from build123d import *

# Parameters (mm, degrees)
F1_DEPTH       = 7
F2_DEPTH       = 6
F3_W           = 4.4
F3_H           = 18
F4_DEPTH       = 18
F6_D           = 4.4
F6_DEPTH       = 5
F6_CSINK_D     = 8.96
F6_CSINK_ANGLE = 90
F6_TIP         = 1.3218933619
F8_DEPTH       = 2.6
F9_R           = 2.2
F10_DEPTH      = 2.3


# Not quite as in the source:
# - a pattern or mirror of a feature is missing from the dataset's text; its kind, count and spacing are read off the source's solid


with BuildPart() as f1:
    # F0 (on Front) → F1 (new body, symmetric)
    with BuildSketch(Plane.XZ):
        with BuildLine():
            Line((129.5, 0), (174.5, 0))
            ThreePointArc((174.5, 0), (174.2671322418, 9.0120264206), (173.5691504848, 18))
            ThreePointArc((173.5691504848, 18), (0, 174.5), (-173.5691504848, 18))
            ThreePointArc((-173.5691504848, 18), (-174.2671322418, 9.0120264206), (-174.5, 0))
            Line((-174.5, 0), (-129.5, 0))
            ThreePointArc((-129.5, 0), (0, 129.5), (129.5, 0))
        make_face()
        with BuildLine():
            ThreePointArc((173.5691504848, 18), (174.2671322418, 9.0120264206), (174.5, 0))
            Line((174.5, 0), (194.5, 0))
            Line((194.5, 0), (194.5, 18))
            Line((194.5, 18), (173.5691504848, 18))
        make_face()
        with BuildLine():
            ThreePointArc((-174.5, 0), (-174.2671322418, 9.0120264206), (-173.5691504848, 18))
            Line((-173.5691504848, 18), (-194.5, 18))
            Line((-194.5, 18), (-194.5, 0))
            Line((-194.5, 0), (-174.5, 0))
        make_face()
    extrude(amount=F1_DEPTH, both=True)

    # F0 (on Front) → F2 (join, symmetric)
    with BuildSketch(Plane.XZ):
        with BuildLine():
            Line((129.5, 0), (174.5, 0))
            ThreePointArc((174.5, 0), (174.2671322418, 9.0120264206), (173.5691504848, 18))
            ThreePointArc((173.5691504848, 18), (0, 174.5), (-173.5691504848, 18))
            ThreePointArc((-173.5691504848, 18), (-174.2671322418, 9.0120264206), (-174.5, 0))
            Line((-174.5, 0), (-129.5, 0))
            ThreePointArc((-129.5, 0), (0, 129.5), (129.5, 0))
        make_face()
        with BuildLine():
            ThreePointArc((173.5691504848, 18), (174.2671322418, 9.0120264206), (174.5, 0))
            Line((174.5, 0), (194.5, 0))
            Line((194.5, 0), (194.5, 18))
            Line((194.5, 18), (173.5691504848, 18))
        make_face()
        with BuildLine():
            ThreePointArc((-174.5, 0), (-174.2671322418, 9.0120264206), (-173.5691504848, 18))
            Line((-173.5691504848, 18), (-194.5, 18))
            Line((-194.5, 18), (-194.5, 0))
            Line((-194.5, 0), (-174.5, 0))
        make_face()
    extrude(amount=F2_DEPTH, both=True)

    # F3 (on face) → F4 (cut)
    with BuildSketch(Plane.YZ.offset(194.5)):
        with Locations((0, 9)):
            Rectangle(F3_W, F3_H)
    f4 = extrude(amount=-F4_DEPTH, mode=Mode.SUBTRACT)

    # F4_copies: F4 across plane
    add(f4.mirror(Plane(origin=(0, 0, 0), x_dir=(0, 0, -1), z_dir=(-1, 0, 0))), mode=Mode.SUBTRACT)

    # F6
    with Locations(Plane.XZ.offset(7)):
        with Locations((185.5, 9)):
            f6 = CounterSinkHole(F6_D / 2, F6_CSINK_D / 2, depth=F6_DEPTH, counter_sink_angle=F6_CSINK_ANGLE)
            with Locations((0, 0, -(F6_DEPTH + F6_TIP / 2))):  # 118° drill point
                Cone(0, F6_D / 2, F6_TIP, mode=Mode.SUBTRACT)

    # F6_copies: F6 across plane
    add(f6.mirror(Plane(origin=(0, 0, 0), x_dir=(0, 0, -1), z_dir=(-1, 0, 0))), mode=Mode.SUBTRACT)

    # F7 (on face) → F8 (cut)
    with BuildSketch(Plane(origin=(0, 7, 0), x_dir=(-1, 0, 0), z_dir=(0, 1, 0))):
        Polygon((-189, 11.0207259422), (-189, 6.9792740578), (-185.5, 4.9585481157), (-182, 6.9792740578), (-182, 11.0207259422), (-185.5, 13.0414518843), align=None)
    f8 = extrude(amount=-F8_DEPTH, mode=Mode.SUBTRACT)

    # F8_copies: F8 across plane
    add(f8.mirror(Plane(origin=(0, 0, 0), x_dir=(0, 0, -1), z_dir=(-1, 0, 0))), mode=Mode.SUBTRACT)

    # F9 (on face) → F10 (cut)
    with BuildSketch(Plane(origin=(0, 4.4, 0), x_dir=(-1, 0, 0), z_dir=(0, 1, 0))):
        with Locations((-185.5, 9)):
            Circle(F9_R)
    f10 = extrude(amount=-F10_DEPTH, mode=Mode.SUBTRACT)

    # F10_copies: F10 across plane
    add(f10.mirror(Plane(origin=(0, 0, 0), x_dir=(0, 0, -1), z_dir=(-1, 0, 0))), mode=Mode.SUBTRACT)


solid = f1.part
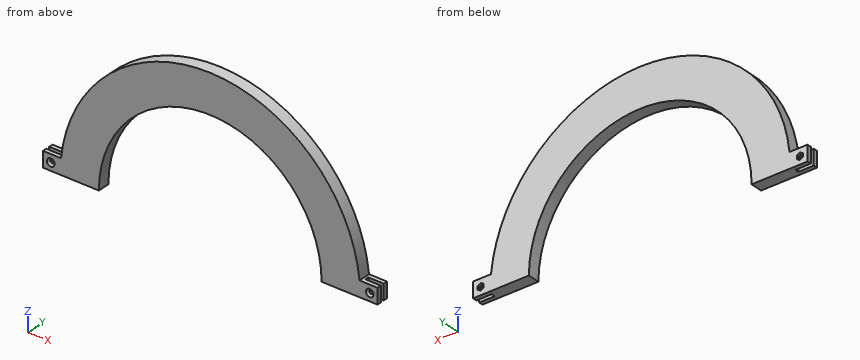
Verification items for the finished model (mm, model axes). Coordinates: 2 decimals unless noted, no trailing zeros. Loops run counter-clockwise (first coordinate to the right, second up) from the corner with the lowest first, then second, coordinate; pieces in that order, holes last. Notation, with made-up numbers: (82.5, 89) -> (120.5, 89) arc R18 cw to (120.5, 100) -> close; hole circle Ø4 at (80.25, -13.5). An arc over 180 degrees is marked (long way). Answer as a JSON object with one key per item and string values. Group by question number.
Item 1: Sectioned sample at B-B on x = 0. Record the boundary of the cut face in (y, z).
Item 2: Depth check by flat-ended pin: pin 1 (2.5 mm diameter, centred on x = 185.5, z = 9, fed in from -Y); pin 2 (8 mm diameter, centred on y = -2.5, z = 55.5, fed in from -X); pin 3 (4 mm diameter, centred on y = 4, z = 79, fed in from -X); pin 4 (5.5 mm diameter, centred on x = 187.5, z = 10.5, fed in from -Y). Enter the tip coordinate at first touch or a pass-through.
Item 3: Sectioned sample at A-A on z = 48.5. Record the boundary of the cut face in (x, y), plus the area to 3 significant figures.
Item 4: Sectioned sample at D-D on x = -76. Record the boundary of the cut face in (y, z).
Item 5: Sectioned sample at C-C on z = 66.5. Record the boundary of the cut face in (x, y).
Item 6: Scan lines: probe 1 along Z at (x, y) = (185.5, -2.9); probe 2 along X at (y, z) = (-3.35, 9); probe 3 along X at (y, z) = (-2, 89). Record each from-to range of solid material in increasing order.
Evaluation:
{
 "1": {"outline": "(-7, 129.5) -> (7, 129.5) -> (7, 174.5) -> (-7, 174.5) -> close"},
 "2": {"pin 1": "passes through", "pin 2": "stops at x = -166.73", "pin 3": "stops at x = -156.59", "pin 4": "stops at y = -7"},
 "3": {"outline": "(-167.62, -7) -> (-120.07, -7) -> (-120.07, 7) -> (-167.62, 7) -> close; (120.07, -7) -> (167.62, -7) -> (167.62, 7) -> (120.07, 7) -> close", "area": "1,330 mm²"},
 "4": {"outline": "(-7, 104.85) -> (7, 104.85) -> (7, 157.08) -> (-7, 157.08) -> close"},
 "5": {"outline": "(-161.33, -7) -> (-111.12, -7) -> (-111.12, 7) -> (-161.33, 7) -> close; (111.12, -7) -> (161.33, -7) -> (161.33, 7) -> (111.12, 7) -> close"},
 "6": {"probe 1": "z = 0 to 6.8, 11.2 to 18", "probe 2": "x = -194.5 to -187.7, -183.3 to -129.19, 129.19 to 183.3, 187.7 to 194.5", "probe 3": "x = -150.1 to -94.07, 94.07 to 150.1"}
}
